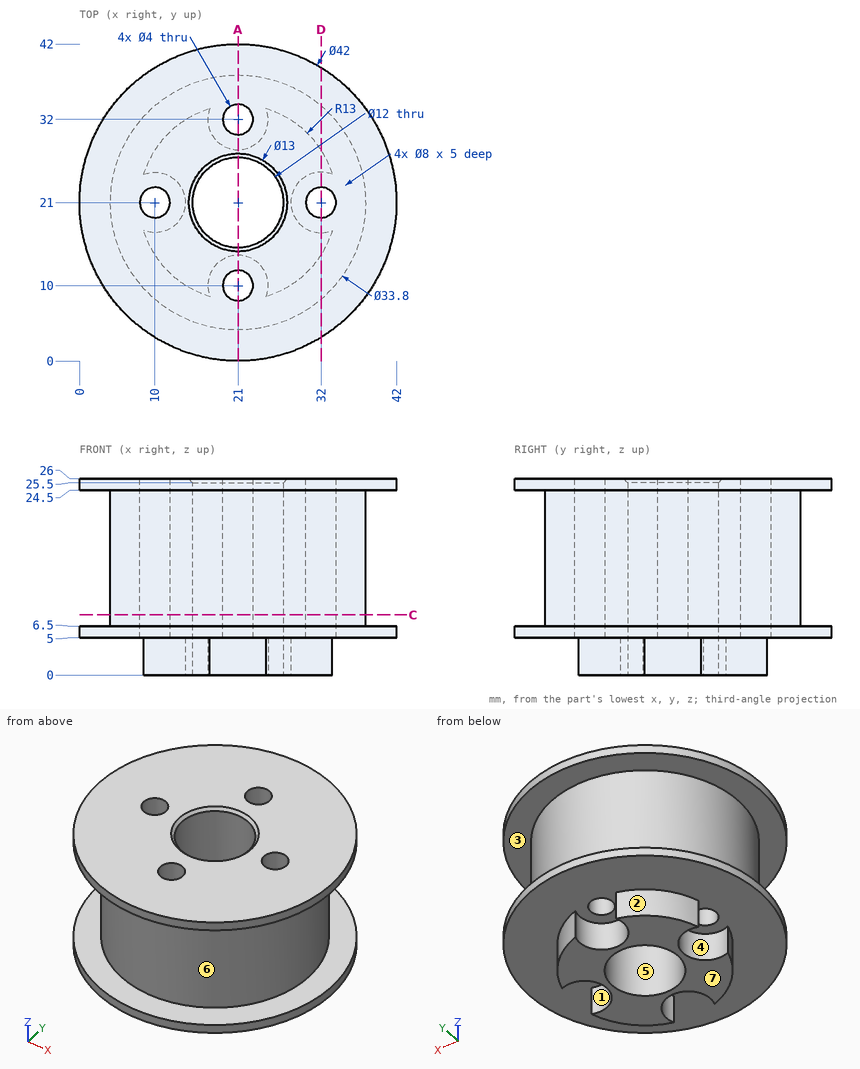
Source: three-view drawing plus pictorial views. Frame: mm from the lowest corner of the part. A direction names the side the tool comes from. Coordinates: 2 decimals unless noted, no trailing zeros. Order: outer loops, then holes, each group sorted by start corner. A loop starts at its lowest first (then second) coordinate and runs counter-clockwise, first axis right, second up. Notation, with made-up numbers: (-6.75, 35.5) -> (46.25, 35.5) arc R18 cw to (46.25, 59.5) -> close; hole circle Ø1 at (-1.75, -24.75). An arc over 180 degrees is marked (long way). Write item = value, one per line.
(1) Access query for the marked faces 1, 2 and 3. Directions: +Z, -Z, +X, -X, +Y, -Y. A direction counts if a zero-diameter tool reaches every point of the face in a straight line with its end or side. Return the directions, or none.
Solved:
face_1 = -Z
face_2 = -Z, -X, +Y
face_3 = none
(2) Pin query (flat end, axial travel): pin 1 Ø3 at (y, z) = (27, 9.5) entering from +X; pin 2 Ø5 at (x, y) = (7, 4.5) entering from -Z; pin 3 Ø5 at (x, z) = (27, 9.5) entering from -Y. Return the tip coordinate at first contact, or that it passes through.
Solved:
pin_1 = 37.29
pin_2 = 5
pin_3 = 4.47
(3) Cut plane C-C on z = 8. Return loops of the section in (x, y), plus the area to 3 significant figures.
Solved:
outline = circle Ø33.8 at (21, 21); hole circle Ø4 at (10, 21); hole circle Ø12 at (21, 21); hole circle Ø4 at (21, 10); hole circle Ø4 at (21, 32); hole circle Ø4 at (32, 21)
area = 734 mm²
(4) Cut plane D-D on x = 32. Return loops of the section in (y, z), plus the area to 3 significant figures.
Solved:
outline = (3.11, 5) -> (14.07, 5) -> (14.07, 0) -> (17, 0) -> (17, 5) -> (19, 5) -> (19, 26) -> (3.11, 26) -> (3.11, 24.5) -> (8.17, 24.5) -> (8.17, 6.5) -> (3.11, 6.5) -> close; (23, 5) -> (25, 5) -> (25, 0) -> (27.93, 0) -> (27.93, 5) -> (38.89, 5) -> (38.89, 6.5) -> (33.83, 6.5) -> (33.83, 24.5) -> (38.89, 24.5) -> (38.89, 26) -> (23, 26) -> close
area = 514 mm²
(5) Line query: line 1 (Z direction, x = 24.5, y = 40.5); line 2 (Y direction, x = 21, z = 3.3); line 3 (Y direction, x = 32, z = 3.5). Output: solid intervals per line, ascending.
Solved:
line_1 = 5 to 6.5, 24.5 to 26
line_2 = 14 to 15, 27 to 28
line_3 = 14.07 to 17, 25 to 27.93
(6) Cut plane A-A on x = 21. Count the separate pieces of the cut face and the enclosed holes in it, plus the area to 3 significant figures.
Solved:
separate_pieces = 4
enclosed_holes = 0
area = 324 mm²
(7) Pull-direction query (X, two-part tool) for the marked faces 4, 5, 6 and 7; classes: pulls with the +X half, pulls with the -X half, needs draft (parallel to the pull), parting line crosses it, or undercut.
Solved:
face_4 = undercut
face_5 = undercut
face_6 = parting line crosses it
face_7 = needs draft
